The listing builds one solid part. Answer for the finished solid, in the listing's coordinates (mm). Round coordinates to 2 decimals unless told otherwise and drop trailing zeros. Write each loop counter-clockwise with the first axis right and the second up, starting at its lowest first coordinate (ties: lowest second). Pieces come first, ordered by that corner, then holes. Notation, with made-up numbers: (29.5, -11.5) - (82.5, -11.5) arc R13 cw to (82.5, 6.5) - close; hole circle Ø5 at (-28.5, 42). An arc over 180 degrees is marked (long way). Use a Markdown table: item, result. Add a question column.
1) Find the intervals of material crossed by probe 1 along Z at (x, y) = (-3.25, -10), in increasing order. Write a range as from..to.
2) A cutting plane is placed at C-C (z = -0.95). Give the vertices of the cut face in (x, y).
3) A cutting plane is placed at D-D (x = 9). Give the vertices of the cut face in (y, z).
4) Determine the mould class of faces 1 (the flat face through (-13.08, 0, 1)), 2 (the flat face through (0, 0, 0)), 3 (the flat face through (0, -12, 1.4)) for opening direction X: +X half, -X half, draft (parallel to the pull), parting line (faces both ways), or undercut.
5) A cutting plane is placed at B-B (x = 2.5). Give the vertices of the cut face in (y, z).
6) A cutting plane is placed at A-A (y = -10.25). Give the vertices of the cut face in (x, z).
7) Each of these flat-tipped pins is pushed along its axis until it touches: P1, Ø1.9, axis at y = -9.5, z = -1, coming from the +X side; P2, Ø1, axis at x = 5.5, z = -1, coming from the +Y side; P3, Ø2, axis at x = 2, y = 9, coming from the -Z side. Where does it stop, or does it pass through?
```python
from build123d import *

# Parameters (mm, degrees)
SKETCH_W     = 26.16
SKETCH_H     = 29.22
PAD_DEPTH    = 1.5
SKETCH001_W  = 23.4
SKETCH001_H  = 23.4
PAD001_DEPTH = 1
SKETCH002_W  = 11.4
SKETCH002_H  = 0.1
PAD002_DEPTH = 1.6
PAD003_DEPTH = 0.1
POCKET_DEPTH = 0.1


with BuildPart() as part:
    # Sketch → Pad (new body)
    with BuildSketch(Plane.XY):
        Rectangle(SKETCH_W, SKETCH_H)
    extrude(amount=PAD_DEPTH)

    # Sketch001 (on Face6 of Pad) → Pad001 (join)
    with BuildSketch(Plane.XY.offset(1.5)):
        with Locations((0, 1.91)):
            Rectangle(SKETCH001_W, SKETCH001_H)
    extrude(amount=-PAD001_DEPTH)

    # Sketch002 (on Face4 of Pad001) → Pad002 (join)
    with BuildSketch(Plane(origin=(0, 0, 0), x_dir=(1, 0, 0), z_dir=(0, 0, -1))):
        with Locations((2.92, 14.56)):
            Rectangle(SKETCH002_W, SKETCH002_H)
    extrude(amount=PAD002_DEPTH)

    # Sketch003 (on Face12 of Pad002) → Pad003 (join)
    with BuildSketch(Plane(origin=(0, 0, -1.6), x_dir=(1, 0, 0), z_dir=(0, 0, -1))):
        with BuildLine():
            Line((-2.78, 14.61), (8.62, 14.61))
            Line((8.62, 14.61), (8.62, 4.248609))
            ThreePointArc((8.12, 3.748609), (8.473553, 3.895055), (8.62, 4.248609))
            Line((8.12, 3.748609), (-2.28, 3.748609))
            ThreePointArc((-2.78, 4.248609), (-2.633553, 3.895055), (-2.28, 3.748609))
            Line((-2.78, 4.248609), (-2.78, 14.61))
        make_face()
    extrude(amount=PAD003_DEPTH)

    # Sketch004 (on Face5 of Pad003) → Pocket (cut)
    with BuildSketch(Plane.XY.offset(1.5)):
        with BuildLine():
            ThreePointArc((-5, -11.81), (-5.5, -12.31), (-5, -12.81))
            Line((-5, -12.81), (5, -12.81))
            ThreePointArc((5, -12.81), (5.5, -12.31), (5, -11.81))
            Line((5, -11.81), (-5, -11.81))
        make_face()
    extrude(amount=-POCKET_DEPTH, mode=Mode.SUBTRACT)


solid = part.part
```
Entries:
| question | item | result |
|---|---|---|
| 1 | probe 1 | z = 0..1.5 |
| 2 | outline | (-2.78, -14.61) - (8.62, -14.61) - (8.62, -14.51) - (-2.78, -14.51) - close |
| 3 | outline | (-14.61, 0) - (14.61, 0) - (14.61, 1.5) - (-14.61, 1.5) - close |
| 4 | face 1 | -X half |
| 4 | face 2 | draft |
| 4 | face 3 | undercut |
| 5 | outline | (-14.61, -1.7) - (-3.75, -1.7) - (-3.75, -1.6) - (-14.51, -1.6) - (-14.51, 0) - (14.61, 0) - (14.61, 1.5) - (-11.81, 1.5) - (-11.81, 1.4) - (-12.81, 1.4) - (-12.81, 1.5) - (-14.61, 1.5) - close |
| 6 | outline | (-13.08, 0) - (13.08, 0) - (13.08, 1.5) - (-13.08, 1.5) - close; (-2.78, -1.7) - (8.62, -1.7) - (8.62, -1.6) - (-2.78, -1.6) - close |
| 7 | P1 | stops at x = 8.62 |
| 7 | P2 | stops at y = -14.51 |
| 7 | P3 | stops at z = 0 |
